Build history of the part. All positions in model axes, mm. Give positions to 0.01 mm unless a question says otherwise; leave off trailing zeros. Write each loop counter-clockwise with the first axis right and the second up, starting at its lowest first coordinate (ties: lowest second). Pieces come first, ordered by that corner, then holes. Notation, with made-up numbers: (75.25, 85) -> (98.25, 85) arc R30 ccw to (98.25, 124) -> close; hole circle Ø11 at (-4.5, -33.75). An arc over 180 degrees is marked (long way). Put each result on its own line as item: value. Start each with the question number.
Item 1: Flat gauge pins, fed straight in: pin 1 Ø6 at (x, y) = (-407.5, 274) entering from +Z; pin 2 Ø6 at (y, z) = (153, 608.5) entering from +X; pin 3 Ø4 at (x, y) = (-390, 194.5) entering from +Z. Where does each tip first touch, or does it go through?
Item 2: Slice it at A-A, the plane y = 95.5. List the corners of the cut face in (x, z), plus the area to 3 significant figures.
Item 3: Drill centre lines: line 1 along X through (y, z) = (220, 616); line 2 along X through (y, z) = (245.5, 646); line 3 along Z through (x, y) = (-145, 84.5). Where is each one in solid material? Low to high.
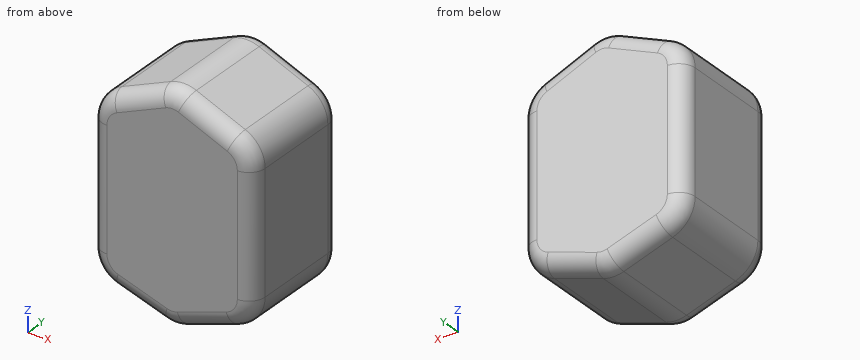
Autodesk Inventor part; units mm, degrees
ref_plane "YZ Plane" through (0, 0, 0) normal (1, 0, 0) x (0, 1, 0)
ref_plane "XZ Plane" through (0, 0, 0) normal (0, 1, 0) x (-1, 0, 0)
ref_plane "XY Plane" through (0, 0, 0) normal (0, 0, 1) x (1, 0, 0)
sketch "Sketch1" plane through (0, 0, 0) normal (0, 1, 0) x (-1, 0, 0)
  line L0 (-8.4597, -4.2821) -> (491.5403, -4.2821)
  line L1 (491.5403, -4.2821) -> (491.5403, 692.7179)
  line L2 (491.5403, 692.7179) -> (-8.4597, 692.7179)
  line L3 (-8.4597, 692.7179) -> (-8.4597, -4.2821)
  point P0 (0, 0)
  dimension "d0" = 500
  dimension "d1" = 697
extrude "Extrusion1" add sketch "Sketch1" along normal blind 372
sketch "Sketch2" plane through (0, 372, 0) normal (0, 1, 0) x (1, 0, 0)
  line L0 (8.4597, 4.2821) -> (-491.5403, 4.2821)
  line L1 (-491.5403, 4.2821) -> (-491.5403, -692.7179)
  line L2 (-491.5403, -692.7179) -> (8.4597, -692.7179)
  line L3 (8.4597, -692.7179) -> (8.4597, 4.2821)
  line L4 (-241.5403, 4.2821) -> (-491.5403, -77.8084)
  line L5 (-241.5403, 4.2821) -> (8.4597, -77.8084)
  line L6 (8.4597, -586.8499) -> (-241.5403, -692.7179)
  line L7 (-241.5403, -692.7179) -> (-491.5403, -586.8499)
  point P0 (0, 0)
extrude "Extrusion2" cut sketch "Sketch2" against normal blind 400 contours L3 L5 L0 | L4 L1 L0 | L3 L2 L6 | L7 L2 L1
fillet "Fillet1" radius 100 6 edges at (-241.5403, 186, 692.7179) (8.4597, 186, 586.8499) (-491.5403, 186, 586.8499) (8.4597, 186, 77.8084) (-241.5403, 186, -4.2821) (-491.5403, 186, 77.8084)
fillet "Fillet2" radius 50 24 edges at (-10.5472, 372, 91.5727) (-135.3429, 372, 30.5891) (-241.5403, 372, 0.971) (-347.7376, 372, 30.5891) (-472.5333, 372, 91.5727) (-491.5403, 372, 335.4127) (-474.9054, 372, 575.8293) (-355.5351, 372, 644.4443) (-241.5403, 372, 684.121) (-127.5454, 372, 644.4443) (-8.1751, 372, 575.8293) (8.4597, 372, 335.4127) (-10.5472, 0, 91.5727) (-135.3429, 0, 30.5891) (-241.5403, 0, 0.971) (-347.7376, 0, 30.5891) (-472.5333, 0, 91.5727) (-491.5403, 0, 335.4127) (-474.9054, 0, 575.8293) (-355.5351, 0, 644.4443) (-241.5403, 0, 684.121) (-127.5454, 0, 644.4443) (-8.1751, 0, 575.8293) (8.4597, 0, 335.4127)
Values follow:
1. pin 1: z = 623.71
1. pin 2: x = -38.7
1. pin 3: z = 630.7
2. outline: (-491.54, 150.23) arc R100 ccw to (-422.74, 55.22) -> (-272.74, 5.96) arc R100 ccw to (-210.34, 5.96) -> (-60.34, 55.22) arc R100 ccw to (8.46, 150.23) -> (8.46, 520.6) arc R100 ccw to (-52.55, 612.68) -> (-202.55, 676.2) arc R100 ccw to (-280.54, 676.2) -> (-430.54, 612.68) arc R100 ccw to (-491.54, 520.6) -> close
2. area: 298,000 mm2
3. line 1: -422.7 to -60.38
3. line 2: -351.86 to -131.22
3. line 3: 27.42 to 651.84
